from build123d import *

# Parameters (mm, degrees)
F0_W          = 88.9
F0_H          = 50.8
F1_DEPTH      = 9.525
F2_W          = 15.875
F2_H          = 19.05
F3_DEPTH      = 6.35
F3_DEPTH_BACK = 22.225
F4_W          = 3.175
F4_H          = 3.175
F5_DEPTH      = 25.4
F5_DEPTH_BACK = 25.4


with BuildPart() as f1:
    # F0 (on Front) → F1 (new body)
    with BuildSketch(Plane.XZ):
        with Locations((1.452832, 0.068092)):
            Rectangle(F0_W, F0_H)
    extrude(amount=F1_DEPTH)

    # F2 (on face) → F3 (join, two sides)
    with BuildSketch(Plane.XZ.offset(9.525)) as f3_sk:
        with Locations((-9.659668, 3.243092)):
            Rectangle(F2_W, F2_H)
    extrude(amount=F3_DEPTH)
    extrude(f3_sk.sketch, amount=-F3_DEPTH_BACK)

    # F4 (on face) → F5 (join, two sides)
    with BuildSketch(Plane.XY.offset(12.768092)) as f5_sk:
        with Locations((-12.834668, 7.9375)):
            Rectangle(F4_W, F4_H)
    extrude(amount=F5_DEPTH)
    extrude(f5_sk.sketch, amount=-F5_DEPTH_BACK)


solid = f1.part
Geometry: final body of the model. Coordinates: model frame, mm. A direction names the side the tool comes from. Coordinates: 2 decimals unless noted, no trailing zeros. Loops run counter-clockwise (first coordinate to the right, second up) from the corner with the lowest first, then second, coordinate; pieces in that order, holes last. Notation, with made-up numbers: (-31.75, 27.5) - (-14.75, 27.5) arc R22 cw to (-14.75, 36.5) - close; hole circle Ø11 at (26, 11.25). An arc over 180 degrees is marked (long way). One line per question, with ' | ' between items. Start each with the question number.
(1) Cut plane C-C on y = 1.5. Output: boundary loops of the cut face in (x, z), and give its area (3 significant figures).
(2) Cut plane A-A on z = -10. Output: boundary loops of the cut face in (x, y) (3 decimals), and give its area (3 significant figures).
(3) Reachability of faces 4 (the flat face through (-10, -13, -6.282)), 5 (the flat face through (-13, 8, -12.632)), 6 (the flat face through (-1.722, -13, 3)), 7 (the flat face through (-11.247, 8, 25)), 8 (the flat face through (-10, -13, 12.768)) from +Z, -Z, +X, -X, +Y, -Y: full face, straight path, thin tool, end or side. Return the list, or none.
(4) Cut plane D-D on x = 18. Output: boundary loops of the cut face in (y, z) (3 decimals).
(5) First-contact query: pin 1 (1.6 mm diameter, centred on x = -13, z = -9, fed in from -Y) (3 decimals); pin 2 (1.6 mm diameter, centred on y = 8.5, z = 27.5, fed in from -X); pin 3 (4 mm diameter, centred on x = 3, y = -2.5, fed in from +Z). Flat tips, straight axial feed; report the tip coordinate or a pass-through.
(6) Draft query along Y for faces 1 (the flat face through (-13, 6.35, 25)), 2 (the flat face through (-13, 9.525, 25)), 3 (the flat face through (-17.597, 6, 3)). Return one class per face: +Y half, -Y half, draft (parallel to the pull), parting line (faces both ways), or undercut.
(7) Cut plane B-B on z = 11. Output: boundary loops of the cut face in (x, y) (3 decimals).
(8) Ray query, L1, parallel to Y at x = 20, z = -9.5 (3 decimals); L2, parallel to Z at x = -0.5, y = -5.25; L3, parallel to X at y = 7, z = 2.5. Return the intervals inside material, ascending. Write a range as from..to.
Here are the results:
1) outline: (-17.6, -6.28) - (-1.72, -6.28) - (-1.72, 12.77) - (-17.6, 12.77) - close | area: 302 mm²
2) outline: (-42.997, -9.525) - (45.903, -9.525) - (45.903, 0) - (-42.997, 0) - close; (-14.422, 6.35) - (-11.247, 6.35) - (-11.247, 9.525) - (-14.422, 9.525) - close | area: 857 mm²
3) face 4: -Z, +X, -X, -Y | face 5: -Z, +X, -X, +Y | face 6: +Z, -Z, +X, -Y | face 7: +Z, +X, +Y | face 8: +Z, +X, -X, -Y
4) outline: (-9.525, -25.332) - (0, -25.332) - (0, 25.468) - (-9.525, 25.468) - close
5) pin 1: y = -9.525 | pin 2: x = -14.42 | pin 3: z = 25.47
6) face 1: undercut | face 2: +Y half | face 3: draft
7) outline: (-42.997, -9.525) - (-17.597, -9.525) - (-17.597, -15.875) - (-1.722, -15.875) - (-1.722, -9.525) - (45.903, -9.525) - (45.903, 0) - (-1.722, 0) - (-1.722, 12.7) - (-17.597, 12.7) - (-17.597, 0) - (-42.997, 0) - close
8) L1: -9.525..0 | L2: -25.33..25.47 | L3: -17.6..-1.72
